For this review, take the finished solid that the model builds, in its own axes (mm). A direction names the side the tool comes from. Coordinates: 2 decimals unless noted, no trailing zeros. Loops run counter-clockwise (first coordinate to the right, second up) from the corner with the lowest first, then second, coordinate; pieces in that order, holes last. Notation, with made-up numbers: (26.5, 42.25) -> (70.5, 42.25) arc R20 cw to (70.5, 73.25) -> close; hole circle Ø2 at (-22.75, 63.5). An arc over 180 degrees is marked (long way). Use a Markdown table: item, result.
from build123d import *

# Parameters (mm, degrees)
SKETCH_5_W          = 100
SKETCH_5_H          = 70
SKETCH_5_R          = 2
EXTRUDE_10_DEPTH    = 0.0001
SKETCH_6_W          = 60
SKETCH_6_H          = 5
EXTRUDE_11_DEPTH    = 45
EXTRUDE_12_DEPTH    = 45
CUT_EXTRUDE_1_DEPTH = 76
SKETCH_16_W         = 16
SKETCH_16_H         = 70
EXTRUDE_16_DEPTH    = 15
CUT_EXTRUDE_2_DEPTH = 49
SKETCH_17_R         = 2
CUT_EXTRUDE_5_DEPTH = 71
FILLET_1_R          = 3
SKETCH_18_W         = 60
SKETCH_18_H         = 65
CUT_EXTRUDE_6_DEPTH = 1.0001
FILLET_2_R          = 4


with BuildPart() as part:
    # Sketch 5 → Extrude 10 (new body)
    with BuildSketch(Plane.XY):
        Rectangle(SKETCH_5_W, SKETCH_5_H)
        with Locations((-41.9, 27)):
            Circle(SKETCH_5_R, mode=Mode.SUBTRACT)
        with Locations((41.9, 27)):
            Circle(SKETCH_5_R, mode=Mode.SUBTRACT)
        with Locations((41.9, -27)):
            Circle(SKETCH_5_R, mode=Mode.SUBTRACT)
        with Locations((-41.9, -27)):
            Circle(SKETCH_5_R, mode=Mode.SUBTRACT)
    extrude(amount=EXTRUDE_10_DEPTH)

    # Sketch 6 → Extrude 11 (add)
    with BuildSketch(Plane.XY.offset(0.0001)):
        with Locations((0, -32.5)):
            Rectangle(SKETCH_6_W, SKETCH_6_H)
    extrude(amount=EXTRUDE_11_DEPTH)

    # Sketch 7 → Extrude 12 (add)
    with BuildSketch(Plane.XY.offset(0.0001)):
        Polygon((-34, -35), (-30, -35), (-30, -30), (-30, 35), (-34, 35), align=None)
        Polygon((34, 35), (30, 35), (30, -30), (30, -35), (34, -35), align=None)
    extrude(amount=EXTRUDE_12_DEPTH)

    # Sketch 8 → Cut-Extrude 1 (cut)
    with BuildSketch(Plane.ZY.offset(34)):
        Polygon((45.0001, -30), (15.0001, 35), (45.0001, 35), align=None)
    extrude(amount=-CUT_EXTRUDE_1_DEPTH, mode=Mode.SUBTRACT)

    # Sketch 16 → Extrude 16 (add)
    with BuildSketch(Plane.XY.offset(0.0001)):
        with Locations((42, 0)):
            Rectangle(SKETCH_16_W, SKETCH_16_H)
        with Locations((-42, 0)):
            Rectangle(SKETCH_16_W, SKETCH_16_H)
    extrude(amount=EXTRUDE_16_DEPTH)

    # Sketch 5_3 → Cut-Extrude 2 (cut)
    with BuildSketch(Plane.XY):
        with BuildLine():
            ThreePointArc((-39.9, 27), (-43.314213562, 28.414213562), (-41.9, 25))
            Line((-41.9, 25), (-41.9, 27))
            Line((-41.9, 27), (-39.9, 27))
        make_face()
        with BuildLine():
            Line((-41.9, 27), (-41.9, 25))
            ThreePointArc((-41.9, 25), (-40.485786438, 25.585786438), (-39.9, 27))
            Line((-39.9, 27), (-41.9, 27))
        make_face()
        with BuildLine():
            ThreePointArc((43.9, 27), (41.9, 29), (39.9, 27))
            Line((39.9, 27), (41.9, 27))
            Line((41.9, 27), (41.9, 25))
            ThreePointArc((41.9, 25), (43.314213562, 25.585786438), (43.9, 27))
        make_face()
        with BuildLine():
            Line((41.9, 27), (39.9, 27))
            ThreePointArc((39.9, 27), (40.485786438, 25.585786438), (41.9, 25))
            Line((41.9, 25), (41.9, 27))
        make_face()
        with BuildLine():
            ThreePointArc((43.9, -27), (43.314213562, -25.585786438), (41.9, -25))
            Line((41.9, -25), (41.9, -27))
            Line((41.9, -27), (39.9, -27))
            ThreePointArc((39.9, -27), (41.9, -29), (43.9, -27))
        make_face()
        with BuildLine():
            Line((41.9, -27), (41.9, -25))
            ThreePointArc((41.9, -25), (40.485786438, -25.585786438), (39.9, -27))
            Line((39.9, -27), (41.9, -27))
        make_face()
        with BuildLine():
            ThreePointArc((-39.9, -27), (-40.485786438, -25.585786438), (-41.9, -25))
            Line((-41.9, -25), (-41.9, -27))
            Line((-41.9, -27), (-39.9, -27))
        make_face()
        with BuildLine():
            Line((-41.9, -27), (-41.9, -25))
            ThreePointArc((-41.9, -25), (-43.314213562, -28.414213562), (-39.9, -27))
            Line((-39.9, -27), (-41.9, -27))
        make_face()
    extrude(amount=CUT_EXTRUDE_2_DEPTH, mode=Mode.SUBTRACT)

    # Sketch 17 → Cut-Extrude 5 (cut, through all)
    with BuildSketch(Plane.XZ.offset(35)):
        with BuildLine():
            Line((0, 22), (-8.485281374, 30.485281374))
            ThreePointArc((-8.485281374, 30.485281374), (-11.08655439, 26.592201188), (-12, 22))
            Line((-12, 22), (0, 22))
        make_face()
        with BuildLine():
            ThreePointArc((0, 34), (-4.592201188, 33.08655439), (-8.485281374, 30.485281374))
            Line((-8.485281374, 30.485281374), (0, 22))
            Line((0, 22), (0, 34))
        make_face()
        with BuildLine():
            Line((8.485281374, 30.485281374), (0, 22))
            Line((0, 22), (8.485281374, 13.514718626))
            ThreePointArc((8.485281374, 13.514718626), (11.08655439, 17.407798812), (12, 22))
            ThreePointArc((12, 22), (11.08655439, 26.592201188), (8.485281374, 30.485281374))
        make_face()
        with BuildLine():
            Line((8.485281374, 13.514718626), (0, 22))
            Line((0, 22), (-8.485281374, 13.514718626))
            ThreePointArc((-8.485281374, 13.514718626), (0, 10), (8.485281374, 13.514718626))
        make_face()
        with BuildLine():
            ThreePointArc((8.485281374, 30.485281374), (4.592201188, 33.08655439), (0, 34))
            Line((0, 34), (0, 22))
            Line((0, 22), (8.485281374, 30.485281374))
        make_face()
        with BuildLine():
            Line((0, 22), (-12, 22))
            ThreePointArc((-12, 22), (-11.08655439, 17.407798812), (-8.485281374, 13.514718626))
            Line((-8.485281374, 13.514718626), (0, 22))
        make_face()
        with Locations((15.5, 6.5)):
            Circle(SKETCH_17_R)
        with Locations((-15.5, 6.5)):
            Circle(SKETCH_17_R)
        with Locations((-15.5, 37.5)):
            Circle(SKETCH_17_R)
        with Locations((15.5, 37.5)):
            Circle(SKETCH_17_R)
    extrude(amount=-CUT_EXTRUDE_5_DEPTH, mode=Mode.SUBTRACT)

    # Fillet 1
    fillet_1_edges = [part.edges().sort_by_distance(p)[0] for p in [
        (34, 0, 15.0001),
        (-34, 0, 15.0001),
        (-34, -32.5, 45.0001),
        (34, -32.5, 45.0001),
    ]]
    fillet(fillet_1_edges, radius=FILLET_1_R)

    # Sketch 18 → Cut-Extrude 6 (cut, through all)
    with BuildSketch(Plane.XY.offset(0.0001)):
        with Locations((0, 2.5)):
            Rectangle(SKETCH_18_W, SKETCH_18_H)
    extrude(amount=-CUT_EXTRUDE_6_DEPTH, mode=Mode.SUBTRACT)

    # Fillet 2
    fillet_2_edges = [part.edges().sort_by_distance(p)[0] for p in [
        (30, -30, 22.50005),
        (-30, -30, 22.50005),
    ]]
    fillet(fillet_2_edges, radius=FILLET_2_R)


solid = part.part
(1) Mouldability with a two-part tool opening along Y and no side actions: class faces 4 (the face through (41.768, 25.004, 7.395)), 5 (the face through (10, -35, 12)), 6 (the face through (-34, -10, 27)), 7 (the face through (-42.334, -28.952, 7.395)) as pulls with the +Y half, pulls with the -Y half, needs draft (parallel to the pull), parting line crosses it, or undercut.
Found:
| item | result |
|---|---|
| face 4 | undercut |
| face 5 | pulls with the -Y half |
| face 6 | needs draft |
| face 7 | undercut |
(2) For faces 1 (the face through (15.066, -32.535, 35.548)), 2 (the face through (43, 0, 15)), 3 (the face through (-6, -30, 33)), list the 3-axis set-ups (+Z, -Z, +X, -X, +Y, -Y) from which the entire face can be reached by the end or side of a thin tool; tool diameter is ignored.
Found:
| item | result |
|---|---|
| face 1 | +Y, -Y |
| face 2 | +Z, +X, +Y, -Y |
| face 3 | +Z, -Z, +Y |
(3) Take a section at C-C on x = -15.5. Write out the cut boundary in (y, z), plus the area to 3 significant figures.
Found:
| item | result |
|---|---|
| outline | (-35, 0) -> (-30, 0) -> (-30, 4.5) -> (-35, 4.5) -> close; (-35, 8.5) -> (-30, 8.5) -> (-30, 35.5) -> (-35, 35.5) -> close; (-35, 39.5) -> (-30, 39.5) -> (-30, 45) -> (-35, 45) -> close |
| area | 185 mm^2 |
(4) Take a section at B-B on y = 18. Write out the cut boundary in (x, z).
Found:
| item | result |
|---|---|
| outline | (-50, 0) -> (-30, 0) -> (-30, 22.85) -> (-34, 22.85) -> (-34, 18) arc R3 cw to (-37, 15) -> (-50, 15) -> close; (30, 0) -> (50, 0) -> (50, 15) -> (37, 15) arc R3 cw to (34, 18) -> (34, 22.85) -> (30, 22.85) -> close |
(5) For pin 1 Ø4 at (x, y) = (45.5, -7.5) entering from +Z; pin 2 Ø6.5 at (x, z) = (15.5, 37.5) entering from +Y; pin 3 Ø10 at (y, z) = (-13.5, 30) entering from +X, all flat-tipped, find the tip position at first contact; note any pin that passes through.
Found:
| item | result |
|---|---|
| pin 1 | stops at z = 15 |
| pin 2 | stops at y = -30 |
| pin 3 | stops at x = 34 |
(6) For line 1 along Z through (x, y) = (-15.5, -33.5); line 2 along X through (y, z) = (-2, 13.5); line 3 along Z through (x, y) = (15, -32), list the stretches that pass through material, from the lowest coordinate up.
Found:
| item | result |
|---|---|
| line 1 | z = 0 to 4.5, 8.5 to 35.5, 39.5 to 45 |
| line 2 | x = -50 to -30, 30 to 50 |
| line 3 | z = 0 to 4.56, 8.44 to 35.56, 39.44 to 45 |
(7) Take a section at D-D on z = 37.5. Write out the cut boundary in (x, y).
Found:
| item | result |
|---|---|
| outline | (-34, -35) -> (-17.5, -35) -> (-17.5, -30) -> (-26, -30) arc R4 cw to (-30, -26) -> (-30, -13.75) -> (-34, -13.75) -> close; (-13.5, -35) -> (13.5, -35) -> (13.5, -30) -> (-13.5, -30) -> close; (17.5, -35) -> (34, -35) -> (34, -13.75) -> (30, -13.75) -> (30, -26) arc R4 cw to (26, -30) -> (17.5, -30) -> close |
